Could you check a few things on this drawing? It's one solid part, dimensions in mm from its lowest x, y, z. Give positions to 0.01 mm unless a question says otherwise; leave off trailing zeros. Loops run counter-clockwise (first coordinate to the right, second up) from the corner with the lowest first, then second, coordinate; pieces in that order, holes last. Notation, with made-up numbers: M 21.5,-20.75 L 46.5,-20.75 A34 ccw 46.5,9.25 Z; hole C 40,61.5 d8. An arc over 180 degrees is marked long. Return JSON: item names as keys, results as strings. Group by question number.
1. For pin 1 (1 mm diameter, centred on x = 1.5, y = 4.5, fed in from -Z); pin 2 (2 mm diameter, centred on y = 3, z = 2, fed in from +X); pin 3 (3 mm diameter, centred on x = 1, z = 4, fed in from +Y), each with a flat end and sliding along its axis, tell me the tip position at first contact or that it passes through.
2. If we section it at B-B (z = 5.25): Write out the boundary of the cut face in (x, y).
3. Please list where these lines run through material, in increasing order: line 1 (Y direction, x = 2.7, z = 3.75); line 2 (Y direction, x = 2, z = 4.75) (1 decimal); line 3 (X direction, y = 4.1, z = 1.25) (1 decimal).
4. If we mould it in two halves opening along Y, with no side actions, what happens to the marked faces 1 and 2? For each: +Y half, -Y half, draft (parallel to the pull), parting line (faces both ways), or undercut.
5. If we section it at A-A (z = 1.75): Write out the boundary of the cut face in (x, y).
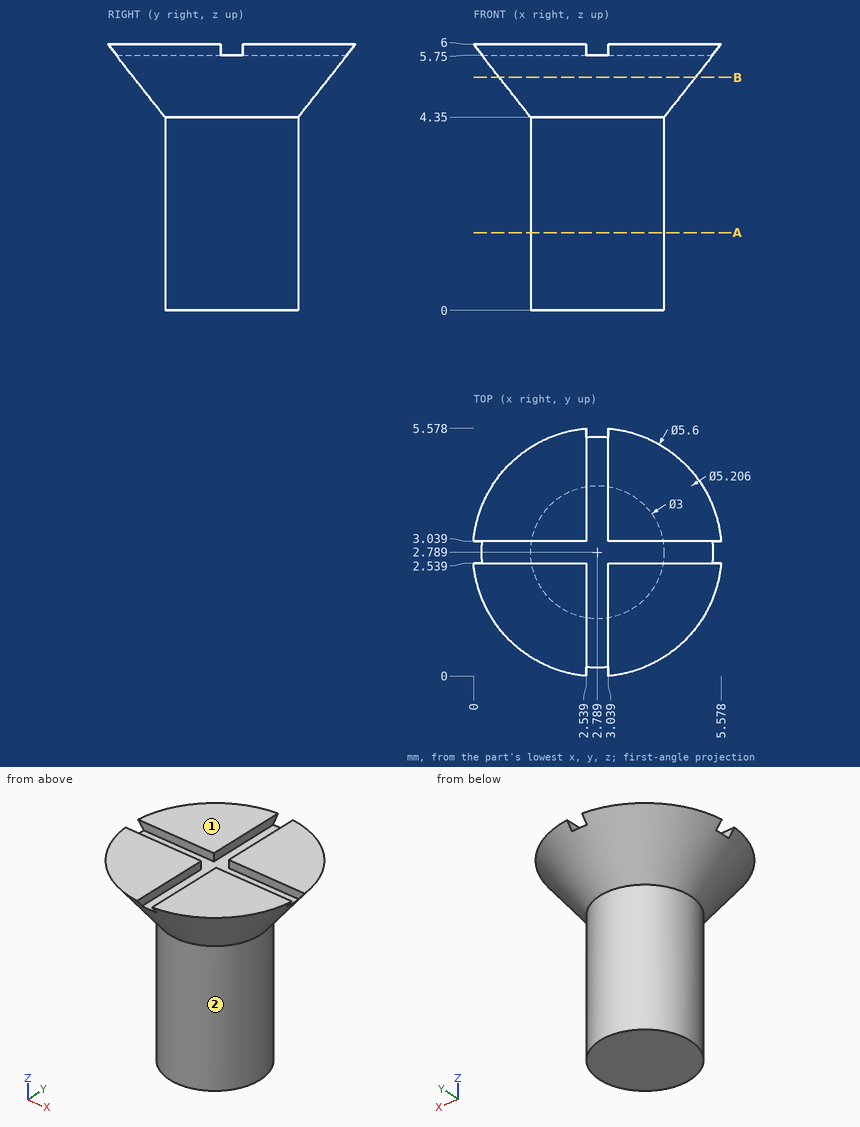
Answer:
{
 "1": {"pin 1": "stops at z = 4.53", "pin 2": "stops at x = 4.29", "pin 3": "stops at y = 4.78"},
 "2": {"outline": "C 2.79,2.79 d4.42"},
 "3": {"line 1": "y = 1.29 to 4.29", "line 2": "y = 1.2 to 4.4", "line 3": "x = 2.1 to 3.5"},
 "4": {"face 1": "draft", "face 2": "parting line"},
 "5": {"outline": "C 2.79,2.79 d3"}
}
